Work out the finished part from the listing and answer in its coordinate system (mm). Face numbers are marked on the shaded views. Coordinates: 2 decimals unless noted, no trailing zeros. Loops run counter-clockwise (first coordinate to the right, second up) from the corner with the lowest first, then second, coordinate; pieces in that order, holes last. Notation, with made-up numbers: (-4.5, 83.5) -> (26.5, 83.5) arc R14 cw to (26.5, 96.5) -> close; hole circle Ø3 at (41, -33). An arc over 180 degrees is marked (long way). Use a Markdown table: item, result.
from build123d import *

# Parameters (mm, degrees)
EXTRUDE_1_DEPTH     = 20
SKETCH_4_W          = 39.68109217
SKETCH_4_H          = 19.592945183
CUT_EXTRUDE_1_DEPTH = 20
SKETCH_7_W          = 132.193091595
SKETCH_7_H          = 30.201739996
CUT_EXTRUDE_2_DEPTH = 20


with BuildPart() as part:
    # 草圖1 → 填料-伸長1 (new body)
    with BuildSketch(Plane(origin=(0, 0, 0), x_dir=(1, 0, 0), z_dir=(0, 1, 0))):
        Polygon((15, -5), (-10, -10), (-15, -10), (-15, 10), (15, 10), align=None)
    extrude(amount=EXTRUDE_1_DEPTH)

    # 草圖4 → 除料-伸長1 (cut)
    with BuildSketch(Plane(origin=(6.101694915, 10.169491525, 10.169491525), x_dir=(0.920574618, -0.276172385, -0.276172385), z_dir=(0.390566733, 0.650944555, 0.650944555))):
        with Locations((1.579314275, 10.72678571)):
            Rectangle(SKETCH_4_W, SKETCH_4_H)
    extrude(amount=CUT_EXTRUDE_1_DEPTH, mode=Mode.SUBTRACT)

    # 草圖7 → 除料-伸長2 (cut)
    with BuildSketch(Plane(origin=(1.016949153, -1.694915254, 1.694915254), x_dir=(-0.920574618, -0.276172385, 0.276172385), z_dir=(-0.390566733, 0.650944555, -0.650944555))):
        with Locations((9.754035329, 10.9182289)):
            Rectangle(SKETCH_7_W, SKETCH_7_H)
    extrude(amount=-CUT_EXTRUDE_2_DEPTH, mode=Mode.SUBTRACT)


solid = part.part
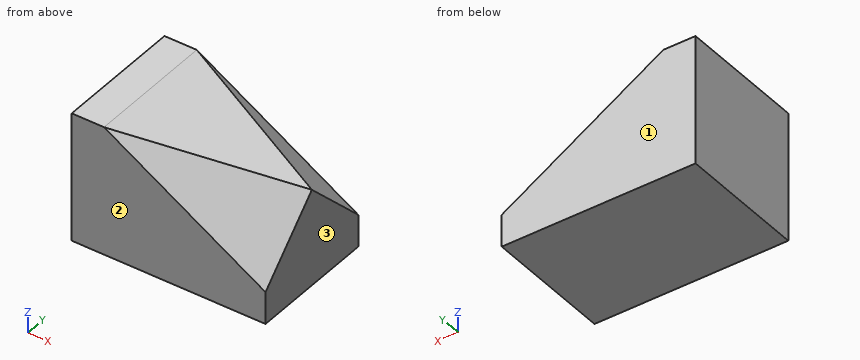
Q1. Given pin 1 Ø4 at (x, y) = (-1.5, 7.5) entering from +Z; pin 2 Ø1 at (x, y) = (-3.5, 9) entering from +Z, each flat-ended and moving along its own axis, determine where each tip first touches the part or whether it passes through.
Solved:
| item | result |
|---|---|
| pin 1 | z = 8.7 |
| pin 2 | z = 8.8 |
Q2. Section B-B on x = 7.5 is taken. Determine the outline of the cut face in (y, z).
Solved:
| item | result |
|---|---|
| outline | (0, -10) -> (20, -10) -> (20, -0.5) -> (13, 6.5) -> (7, 6.5) -> (0, -0.5) -> close |
Q3. Section A-A on y = 2.5 is taken. Determine the outline of the cut face in (x, z), and give its area (3 significant figures).
Solved:
| item | result |
|---|---|
| outline | (-15, -10) -> (15, -10) -> (15, -2.5) -> (-3.75, 8.75) -> (-10, 10) -> (-15, 10) -> close |
| area | 467 mm² |
Q4. Determine the mould class of the marked faces 1, 2 and 3 for opening direction Y: pulls with the +Y half, pulls with the -Y half, needs draft (parallel to the pull), parting line crosses it, or undercut.
Solved:
| item | result |
|---|---|
| face 1 | pulls with the +Y half |
| face 2 | pulls with the -Y half |
| face 3 | needs draft |
Q5. Consider line 1 (Z direction, x = 5, y = 2); line 2 (Z direction, x = 12, y = 9); line 3 (X direction, y = 2.25, z = 8.25). Determine where each line is inside the solid, lowest interval first. Write a range as [from, to].
Solved:
| item | result |
|---|---|
| line 1 | [-10, 3] |
| line 2 | [-10, 5.6] |
| line 3 | [-15, -3.33] |
